Read the model definition and answer for the solid it produces. Units are mm, in the model's axes. A direction names the side the tool comes from. Coordinates: 2 decimals unless noted, no trailing zeros. Order: outer loops, then holes, each group sorted by start corner. A loop starts at its lowest first (then second) coordinate and runs counter-clockwise, first axis right, second up. Notation, with made-up numbers: M 23.5,-19.75 L 77.5,-19.75 A20 ccw 77.5,18.25 Z; hole C 82.25,53.25 d1. An arc over 180 degrees is marked long. Put each result on its own line as item: value.
from build123d import *

# Parameters (mm, degrees)
SKETCH1_R           = 2.3
SKETCH1_R_2         = 10.75
BOSS_EXTRUDE1_DEPTH = 6.35


with BuildPart() as part:
    # Sketch1 → Boss-Extrude1 (new body)
    with BuildSketch(Plane.XY):
        Polygon((-1, 138), (341, 138), (341, 6), (27, 6), (27, 10.7), (3.7, 10.7), (3.7, 33), (-1, 33), align=None)
        with Locations((276, 112.7)):
            Circle(SKETCH1_R, mode=Mode.SUBTRACT)
        with Locations((276, 29.5)):
            Circle(SKETCH1_R, mode=Mode.SUBTRACT)
        with Locations((196, 87.7)):
            Circle(SKETCH1_R_2, mode=Mode.SUBTRACT)
        Polygon((293.7, 35), (252.7, 35), (252.7, 54), (258.3, 54), (258.3, 109), (293.7, 109), align=None, mode=Mode.SUBTRACT)
    extrude(amount=BOSS_EXTRUDE1_DEPTH)


solid = part.part
Q1. A tool of negligible diameter and unlimited length cuts with its end or side. For faces 1 (the face through (341, 73, 3)), 2 (the face through (276, 109, 3)), 3 (the face through (16, 10.7, 3)), from which of +Z, -Z, +X, -X, +Y, -Y can it reach the whole face along a straight path? Write none if from no direction.
Answers below:
face 1: +Z, -Z, +X, +Y, -Y
face 2: +Z, -Z
face 3: +Z, -Z, -X, -Y
Q2. Consider line 1 along Y through (x, z) = (276, 1.75); line 2 along X through (y, z) = (91, 1.75); line 3 along X through (y, z) = (63, 4.75). Determine where each line is inside the solid, lowest interval first.
Answers below:
line 1: y = 6 to 27.2, 31.8 to 35, 109 to 110.4, 115 to 138
line 2: x = -1 to 185.77, 206.23 to 258.3, 293.7 to 341
line 3: x = -1 to 258.3, 293.7 to 341
Q3. For a pull along X with two mould halves and no side action, classify faces 4 (the face through (172, 73, 6.35)), 5 (the face through (273, 35, 3)), 6 (the face through (-1, 85, 3)), 7 (the face through (252.7, 44, 3)) as +X half, -X half, draft (parallel to the pull), parting line (faces both ways), or undercut.
Answers below:
face 4: draft
face 5: undercut
face 6: -X half
face 7: undercut
Q4. Find section B-B on z = 2.5. Write down the section's boundary in (x, y).
Answers below:
outline: M -1,33 L 3.7,33 L 3.7,10.7 L 27,10.7 L 27,6 L 341,6 L 341,138 L -1,138 Z; hole C 196,87.7 d21.5; hole M 252.7,35 L 293.7,35 L 293.7,109 L 258.3,109 L 258.3,54 L 252.7,54 Z; hole C 276,29.5 d4.6; hole C 276,112.7 d4.6
Q5. Given pin 1 (3 mm diameter, centred on x = 276, y = 112.7, fed in from +Z); pin 2 (1 mm diameter, centred on x = 170, y = 89, fed in from -Z), each flat-ended and moving along its own axis, determine where each tip first touches the part or whether it passes through.
Answers below:
pin 1: passes through
pin 2: stops at z = 0
Q6. Find section A-A on y = 44. Write down the section's boundary in (x, z), plus the area to 3 significant figures.
Answers below:
outline: M -1,0 L 252.7,0 L 252.7,6.35 L -1,6.35 Z; M 293.7,0 L 341,0 L 341,6.35 L 293.7,6.35 Z
area: 1,910 mm^2
Q7. Find section D-D on y = 87.7. Write down the section's boundary in (x, z), plus the area to 3 significant figures.
Answers below:
outline: M -1,0 L 185.25,0 L 185.25,6.35 L -1,6.35 Z; M 206.75,0 L 258.3,0 L 258.3,6.35 L 206.75,6.35 Z; M 293.7,0 L 341,0 L 341,6.35 L 293.7,6.35 Z
area: 1,810 mm^2
Q8. Find section C-C on x = 196. Write down the section's boundary in (y, z), plus the area to 3 significant figures.
Answers below:
outline: M 6,0 L 76.95,0 L 76.95,6.35 L 6,6.35 Z; M 98.45,0 L 138,0 L 138,6.35 L 98.45,6.35 Z
area: 702 mm^2
